from build123d import *

# Parameters (mm, degrees)
BOSS_EXTRUDE1_DEPTH = 25
CUT_EXTRUDE3_START  = -25
SKETCH5_R           = 4.4
CUT_EXTRUDE3_DEPTH  = 4.8
SKETCH6_OUTSIDE_W   = 108.03
SKETCH6_OUTSIDE_H   = 47.53
CUT_EXTRUDE4_DEPTH  = 25
SKETCH8_W           = 50.5
SKETCH8_H           = 25.070079704
CUT_EXTRUDE5_DEPTH  = 3.5


with BuildPart() as part:
    # Sketch2 → Boss-Extrude1 (new body)
    with BuildSketch(Plane.XY):
        with BuildLine():
            Line((53.900497512, 28.014925373), (27.014667046, 28.014925373))
            ThreePointArc((27.014667046, 28.014925373), (25.389308303, 27.180347595), (25.120437848, 25.373134328))
            ThreePointArc((25.120437848, 25.373134328), (11.150497512, 5.889925373), (-2.819442823, 25.373134328))
            ThreePointArc((-2.819442823, 25.373134328), (-3.088313278, 27.180347595), (-4.713672021, 28.014925373))
            Line((-4.713672021, 28.014925373), (-31.599502488, 28.014925373))
            Line((-31.599502488, 28.014925373), (-31.599502488, -22.985074627))
            Line((-31.599502488, -22.985074627), (53.900497512, -22.985074627))
            Line((53.900497512, -22.985074627), (53.900497512, 28.014925373))
        make_face()
    extrude(amount=BOSS_EXTRUDE1_DEPTH)

    # Sketch5 → Cut-Extrude3 (cut)
    with BuildSketch(Plane.XY.offset(25).offset(CUT_EXTRUDE3_START)):
        with Locations((11.150497512, -2.910074627)):
            Circle(SKETCH5_R)
    extrude(amount=CUT_EXTRUDE3_DEPTH, mode=Mode.SUBTRACT)

    # Sketch6 outside → Cut-Extrude4 (cut)
    with BuildSketch(Plane(origin=(0, 28.014925373, 0), x_dir=(1, 0, 0), z_dir=(0, 1, 0))):
        with Locations((11.15, -12.5)):
            Rectangle(SKETCH6_OUTSIDE_W, SKETCH6_OUTSIDE_H)
        Polygon((-24.599502488, 0), (-26.73851519, -7.13632431), (-14.574659319, -7.13632431), (-16.713672021, 0), (-4.713672021, 0), (27.014667046, 0), (39.014667046, 0), (36.875076634, -7.136151124), (49.040087925, -7.136151124), (46.900497512, 0), (53.900497512, 0), (53.900497512, -25), (46.900497512, -25), (49.040087925, -17.863848876), (36.875076634, -17.863848876), (39.014667046, -25), (27.014667046, -25), (-4.713672021, -25), (-16.713672021, -25), (-14.574081609, -17.863848876), (-26.7390929, -17.863848876), (-24.599502488, -25), (-31.599502488, -25), (-31.599502488, 0), align=None, mode=Mode.SUBTRACT)
    extrude(amount=-CUT_EXTRUDE4_DEPTH, mode=Mode.SUBTRACT)

    # Sketch8 → Cut-Extrude5 (cut)
    with BuildSketch(Plane(origin=(0, 0, 2.5), x_dir=(-1, 0, 0), z_dir=(0, 0, -1))):
        with Locations((-11.150497512, 15.479885521)):
            Rectangle(SKETCH8_W, SKETCH8_H)
    extrude(amount=-CUT_EXTRUDE5_DEPTH, mode=Mode.SUBTRACT)


solid = part.part
Build history of the part. All positions in model axes, mm. A direction names the side the tool comes from. Give positions to 0.01 mm unless a question says otherwise; leave off trailing zeros. Loops run counter-clockwise (first coordinate to the right, second up) from the corner with the lowest first, then second, coordinate; pieces in that order, holes last. Notation, with made-up numbers: (6, 32.25) -> (11, 32.25) arc R24 ccw to (11, 63.25) -> close; hole circle Ø7 at (8.5, 7.5). An arc over 180 degrees is marked (long way). Answer in a Markdown table with one row per item.
Item 1: Probe line 1 along X through (y, z) = (21, 19.75); line 2 along Z through (x, y) = (-7, 24.5); line 3 along X through (y, z) = (14.5, 19.75). List the from-to ranges inside material, lowest first. Write a range as [from, to].
Findings below:
| item | result |
|---|---|
| line 1 | x = [-31.6, -26.17], [-15.14, -3.6], [25.9, 37.44], [48.47, 53.9] |
| line 2 | z = [0, 2.5], [6, 25] |
| line 3 | x = [-31.6, -26.17], [-15.14, -2.26], [24.56, 37.44], [48.47, 53.9] |
Item 2: Mould opens along Z. For faces 4 (the flat face through (47.985, 15.69, 3.618)), 5 (the cylindrical face through (6.755, -2.717, 2.366)) say: pulls with the +Z half, pulls with the -Z half, needs draft (parallel to the pull), parting line crosses it, or undercut.
Findings below:
| item | result |
|---|---|
| face 4 | undercut |
| face 5 | needs draft |
Item 3: Slice it at C-C on z = 13.5. Write the cut outline in (x, y), plus the area to 3 significant figures.
Findings below:
| item | result |
|---|---|
| outline | (-31.6, -22.99) -> (53.9, -22.99) -> (53.9, 28.01) -> (27.01, 28.01) arc R2 ccw to (25.12, 25.37) arc R14.75 cw (long way) to (-2.82, 25.37) arc R2 ccw to (-4.71, 28.01) -> (-31.6, 28.01) -> close |
| area | 3,810 mm² |
Item 4: Slice it at D-D on x = 12. Write the cut outline in (y, z).
Findings below:
| item | result |
|---|---|
| outline | (-22.99, 0) -> (-7.23, 0) -> (-7.23, 4.8) -> (1.41, 4.8) -> (1.41, 0) -> (5.91, 0) -> (5.91, 2.5) -> (2.94, 2.5) -> (2.94, 6) -> (5.91, 6) -> (5.91, 25) -> (-22.99, 25) -> close |
Item 5: Slice it at B-B on x = -23. Write the cut outline in (y, z).
Findings below:
| item | result |
|---|---|
| outline | (-22.99, 0) -> (3.01, 0) -> (3.01, 7.14) -> (28.01, 7.14) -> (28.01, 17.86) -> (3.01, 17.86) -> (3.01, 25) -> (-22.99, 25) -> close |
Item 6: Tool access for faces 1 (the flat face through (-21, 3.015, 4)), 2 (the flat face through (-18, 28.015, 12)), 3 (the cylindrical face through (-3.073, 27.159, 15.367)): list every direction of +Z, -Z, +X, -X, +Y, -Y with a clear straight run to the whole face (end or side of a thin tool).
Findings below:
| item | result |
|---|---|
| face 1 | +Y |
| face 2 | +Z, -Z, +X, -X, +Y |
| face 3 | +Z, -Z |
Item 7: Flat gauge pins, fed straight in: P1, Ø3.5, axis at x = -18.5, z = 23, coming from the +Y side; P2, Ø2.5, axis at x = 12, y = -4, coming from the -Z side; P3, Ø4, axis at x = -0.5, z = 5, coming from the +Y side. Where does each tip first touch, or does it go through?
Findings below:
| item | result |
|---|---|
| P1 | stops at y = 3.01 |
| P2 | stops at z = 4.8 |
| P3 | stops at y = 14.44 |
